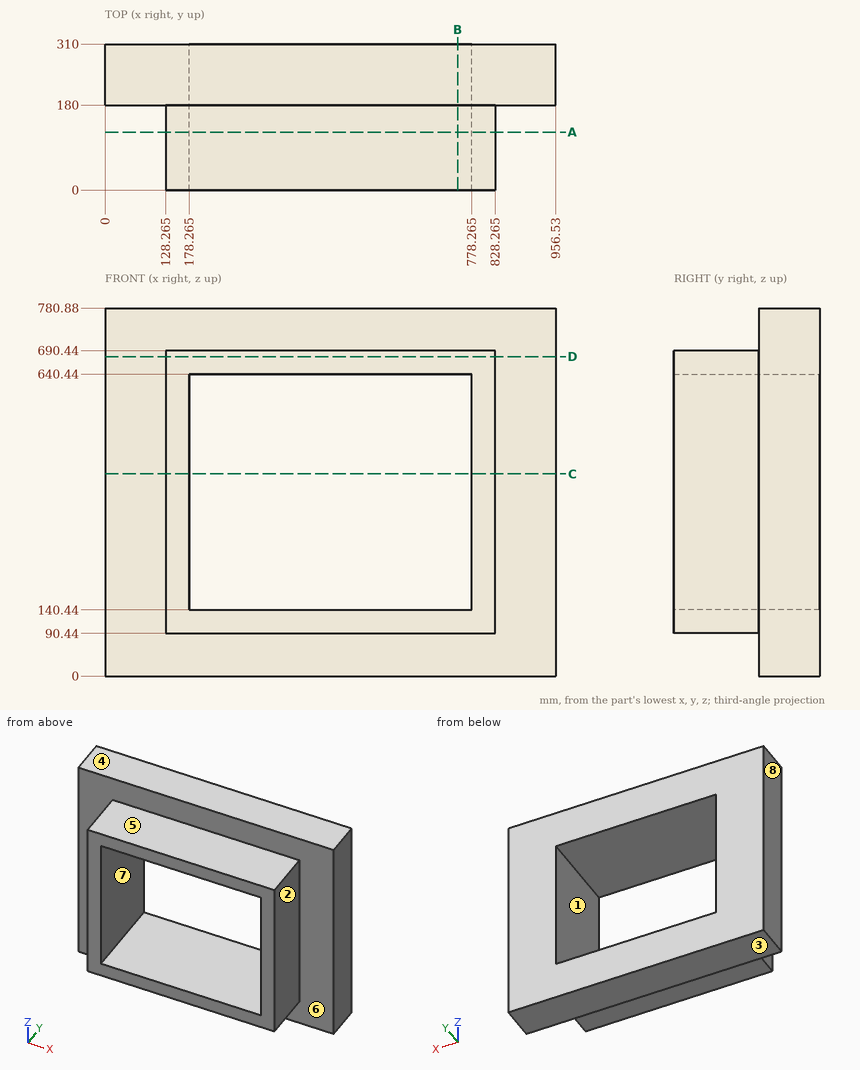
Design review of the part shown in the three views and the two pictorial views. Dimensions are in mm from the part's minimum x, y and z. A direction names the side the tool comes from. Round coordinates to 2 decimals unless told otherwise and drop trailing zeros. Loops run counter-clockwise (first coordinate to the right, second up) from the corner with the lowest first, then second, coordinate; pieces in that order, holes last. Notation, with made-up numbers: (88.25, -16.75) - (108.25, -16.75) arc R22 cw to (108.25, 7.25) - close; hole circle Ø4 at (54.25, -15). An arc over 180 degrees is marked (long way). One line per item, written item: value. Start each with the question number.
Item 1: Take a section at C-C (z = 429). Give the boundary of the cut face in (x, y) (3 decimals), plus the area to 3 significant figures.
Item 2: For L1, parallel to Z at x = 696, y = 75.5; L2, parallel to X at y = 76.5, z = 636.5 (3 decimals); L3, parallel to Z at x = 504, y = 270, list the stretches that pass through material, from the lowest coordinate up.
Item 3: The part is to be moulded in two halves that separate along X. For the marked faces 6, 7 and 8, say which applies: +X half, -X half, draft (parallel to the pull), parting line (faces both ways), or undercut.
Item 4: Take a section at B-B (x = 748). Give the boundary of the cut face in (y, z), plus the area to 3 significant figures.
Item 5: Take a section at D-D (z = 678). Give the boundary of the cut face in (x, y) (3 decimals), plus the area to 3 significant figures.
Item 6: Take a section at A-A (y = 123). Give the boundary of the cut face in (x, z) (3 decimals), plus the area to 3 significant figures.
Item 7: For the marked faces 1, 2, 3, 4 and 5, list the 3-axis set-ups (+Z, -Z, +X, -X, +Y, -Y) from which the entire face can be reached by the end or side of a thin tool; tool diameter is ignored.
Item 8: Clearance check with a flat-ended pin moving along its axis: pin 1 Ø1.5 at (y, z) = (168, 638.5) entering from +X (3 decimals). State where the tip first meets the part, or that it passes through.
Answer below:
1. outline: (0, 180) - (128.265, 180) - (128.265, 0) - (178.265, 0) - (178.265, 310) - (0, 310) - close; (778.265, 0) - (828.265, 0) - (828.265, 180) - (956.53, 180) - (956.53, 310) - (778.265, 310) - close
1. area: 64,300 mm2
2. L1: z = 90.44 to 140.44, 640.44 to 690.44
2. L2: x = 128.265 to 178.265, 778.265 to 828.265
2. L3: z = 0 to 140.44, 640.44 to 780.88
3. face 6: draft
3. face 7: undercut
3. face 8: -X half
4. outline: (0, 90.44) - (180, 90.44) - (180, 0) - (310, 0) - (310, 140.44) - (0, 140.44) - close; (0, 640.44) - (310, 640.44) - (310, 780.88) - (180, 780.88) - (180, 690.44) - (0, 690.44) - close
4. area: 54,500 mm2
5. outline: (0, 180) - (128.265, 180) - (128.265, 0) - (828.265, 0) - (828.265, 180) - (956.53, 180) - (956.53, 310) - (0, 310) - close
5. area: 250,000 mm2
6. outline: (128.265, 90.44) - (828.265, 90.44) - (828.265, 690.44) - (128.265, 690.44) - close; hole (178.265, 140.44) - (778.265, 140.44) - (778.265, 640.44) - (178.265, 640.44) - close
6. area: 120,000 mm2
7. face 1: +Y, -Y
7. face 2: +Z, -Z, +X, -Y
7. face 3: -Z, +X, -X, +Y, -Y
7. face 4: +Z, +X, -X, +Y, -Y
7. face 5: +Z, +X, -X, -Y
8. pin 1: stops at x = 828.265
